Autodesk Fusion 360 part; units mm, degrees
sketch "Sketch1" plane through (0, 0, 0) normal (0, 1, 0) x (1, 0, 0)
  circle A0 centre (0, 0) radius 30
  dimension "d1" = 60
extrude "Extrude1" add sketch "Sketch1" against normal blind 10
sketch "Sketch2" plane through (0, -10, 0) normal (0, -1, 0) x (1, 0, 0)
  circle A0 centre (0, 0) radius 30
  line L0 (0, -30) -> (-80, -30)
  line L1 (-80, -30) -> (-80, -20)
  line L2 (-80, -20) -> (0, -20)
  line L3 (0, -20) -> (0, -30)
  dimension "d4" = 80
  dimension "d5" = 10
extrude "Extrude2" add sketch "Sketch2" against normal blind 70 contours A0 L0 L1 L2 | A0 L2 L3 picked at (-1.3972, -26.5686)
sketch "Sketch3" plane through (-80, 0, 0) normal (-1, 0, 0) x (0, -1, 0)
  line L0 (10, -30) -> (10, -20)
  line L1 (10, -20) -> (-60, -20)
  line L2 (-60, -20) -> (-60, -30)
  line L3 (-60, -30) -> (10, -30)
  circle A0 centre (-25, 0) radius 30
  line L4 (-25, 0) -> (-25, -30) construction
  dimension "d8" = 60
extrude "Extrude3" add sketch "Sketch3" against normal blind 10 contours L1 A0 picked at (-17.2718, 11.3343)
sketch "Sketch4" plane through (0, 0, 0) normal (0, 1, 0) x (-1, 0, 0)
  line L0 (0, -30) -> (0, -20)
  line L1 (0, -20) -> (22.3607, -20)
  arc A0 (22.3607, -20) -> (0, -30) centre (0, 0) ccw
  line L2 (-15.5, 15.5) -> (15.5, 15.5)
  line L3 (15.5, 15.5) -> (15.5, -15.5)
  line L4 (15.5, -15.5) -> (-15.5, -15.5)
  line L5 (-15.5, -15.5) -> (-15.5, 15.5)
  line L6 (-15.5, 15.5) -> (15.5, -15.5) construction
  line L7 (15.5, 15.5) -> (-15.5, -15.5) construction
  dimension "d11" = 31
  dimension "d12" = 31
hole "Hole1" at (15.5, 0, 15.5) at (-15.5, 0, 15.5) at (15.5, 0, -15.5) at (-15.5, 0, -15.5) direction (0, -1, 0) diameter 2.529 depth 10 tip angle 118
hole "Hole2" at (0, 0, 0) direction (0, -1, 0) diameter 6 depth 10 tip angle 118
sketch "Sketch5" plane through (-70, 0, 0) normal (1, 0, 0) x (0, 1, 0)
  arc A0 (47.3607, -20) -> (2.6393, -20) centre (25, 0) ccw
  line L0 (2.6393, -20) -> (47.3607, -20)
  line L1 (9.5, 15.5) -> (40.5, 15.5)
  line L2 (40.5, 15.5) -> (40.5, -15.5)
  line L3 (40.5, -15.5) -> (9.5, -15.5)
  line L4 (9.5, -15.5) -> (9.5, 15.5)
  line L5 (9.5, 15.5) -> (40.5, -15.5) construction
  line L6 (40.5, 15.5) -> (9.5, -15.5) construction
  point P0 (25, 0)
  dimension "d21" = 31
  dimension "d22" = 31
hole "Hole3" at (-70, 9.5, 15.5) at (-70, 40.5, 15.5) at (-70, 9.5, -15.5) at (-70, 40.5, -15.5) direction (-1, 0, 0) diameter 2.529 depth 10 tip angle 118
hole "Hole4" at (-70, 25, 0) direction (-1, 0, 0) diameter 6 depth 10 tip angle 118
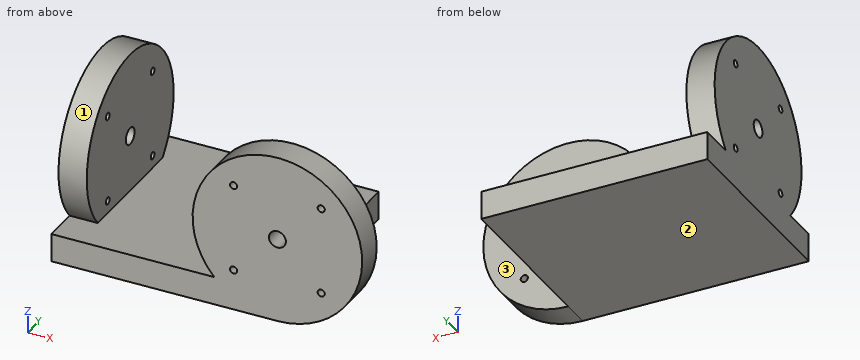
Geometry check sheet. Reference: the model listing, model coordinates, mm. Face numbers are marked on the shaded views. Round coordinates to 2 decimals unless told otherwise and drop trailing zeros. Write each loop counter-clockwise with the first axis right and the second up, starting at its lowest first coordinate (ties: lowest second). Pieces come first, ordered by that corner, then holes. Notation, with made-up numbers: (-31, -37.75) -> (-16, -37.75) arc R34 cw to (-16, -0.75) -> close; hole circle Ø10 at (83.25, 80). An arc over 180 degrees is marked (long way). Put each result on its own line as item: value.
1) Cross-section at C-C, the plane y = 9.5. Enter the section's corners in (x, z), plus the area to 3 significant figures.
Recorded:
outline: (-80, -30) -> (0, -30) -> (0, -20) -> (-70, -20) -> (-70, -16.76) -> (-80, -16.76) -> close; (-80, -14.24) -> (-70, -14.24) -> (-70, 14.24) -> (-80, 14.24) -> close; (-80, 16.76) -> (-70, 16.76) -> (-70, 25.69) -> (-80, 25.69) -> close
area: 1,210 mm2
2) Cross-section at B-B, the plane z = 0. Enter the section's corners in (x, y).
Recorded:
outline: (-80, -5) -> (-70, -5) -> (-70, 22) -> (-80, 22) -> close; (-80, 28) -> (-70, 28) -> (-70, 55) -> (-80, 55) -> close; (-30, -10) -> (-3, -10) -> (-3, 0) -> (-30, 0) -> close; (3, -10) -> (30, -10) -> (30, 0) -> (3, 0) -> close
3) Cross-section at D-D, the plane x = -15.5. Enter the section's corners in (y, z).
Recorded:
outline: (-10, -30) -> (60, -30) -> (60, -20) -> (0, -20) -> (0, -16.76) -> (-10, -16.76) -> close; (-10, -14.24) -> (0, -14.24) -> (0, 14.24) -> (-10, 14.24) -> close; (-10, 16.76) -> (0, 16.76) -> (0, 25.69) -> (-10, 25.69) -> close
4) Thickness scan on probe 1 along X at (y, z) = (-6.25, 15.5); probe 2 along Y at (x, z) = (-73.75, 15.5); probe 3 along Z at (x, y) = (-46.5, 33). Record the ranges inside material, lowest first. Write a range as from..to.
Recorded:
probe 1: x = -25.69..-16.76, -14.24..14.24, 16.76..25.69
probe 2: y = -0.69..8.24, 10.76..39.24, 41.76..50.69
probe 3: z = -30..-20
5) Cross-section at A-A, the plane z = 24. Enter the section's corners in (x, y).
Recorded:
outline: (-80, 7) -> (-70, 7) -> (-70, 43) -> (-80, 43) -> close; (-18, -10) -> (18, -10) -> (18, 0) -> (-18, 0) -> close
6) Depth check by flat-ended pin: P1, Ø8, axis at x = 0, z = 0, coming from the +Y side; P2, Ø1, axis at x = -26, y = 30, coming from the +Z side; P3, Ø11, axis at y = 36, z = -24.5, coming from the +X side. Enter the tip coordinate at first touch or a pass-through.
Recorded:
P1: stops at y = 0
P2: stops at z = -20
P3: stops at x = 0
7) Release check for a two-part mould opening along Z. For the marked faces 1, 2 and 3 record: pulls with the +Z half, pulls with the -Z half, needs draft (parallel to the pull), parting line crosses it, or undercut.
Recorded:
face 1: undercut
face 2: pulls with the -Z half
face 3: needs draft
